Part model, mm, in its own coordinate system. Face numbers are marked on the shaded views. A direction names the side the tool comes from. Coordinates: 2 decimals unless noted, no trailing zeros. Order: outer loops, then holes, each group sorted by start corner. A loop starts at its lowest first (then second) coordinate and runs counter-clockwise, first axis right, second up.
1) Mould opens along X. For the marked faces 1, 2 and 3 say: +X half, -X half, draft (parallel to the pull), parting line (faces both ways), or undercut.
2) Cut at A-A (y = 8.25). List the corners of the cut face in (x, z), and give its area (3 significant figures).
3) Pin check, flat tips, straight feed: pin 1 Ø3 at (y, z) = (4.5, 7) entering from +X; pin 2 Ø3.5 at (x, z) = (-1, -1.5) entering from -Y; pin 3 Ø2 at (x, z) = (-3, 5) entering from -Y. Stop position of each tip, or through.
4) Wall check: L1, parallel to X at y = 13.75, z = 0; L2, parallel to Y at x = -7, z = 3.5; L3, parallel to Y at x = -7.75, z = -1.5. Give the ranges that are in metal, low to high.
5) Tool access for the marked faces 4 and 5: list every direction of +Z, -Z, +X, -X, +Y, -Y with a clear straight run to the whole face (end or side of a thin tool).
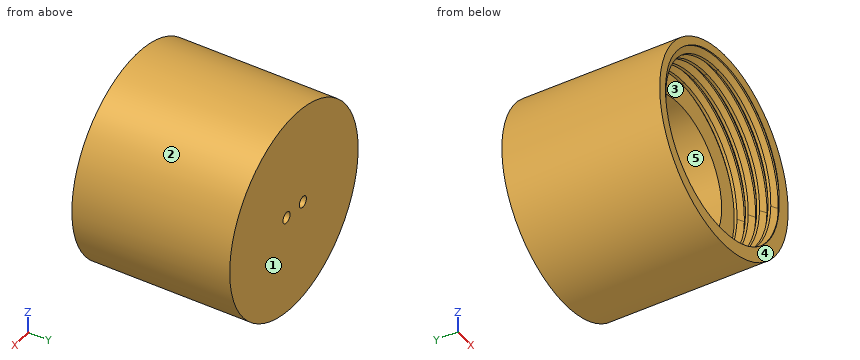
```python
from build123d import *

# Parameters (mm, degrees)
SKETCH1_R           = 9
SKETCH1_R_2         = 7.75
BOSS_EXTRUDE1_DEPTH = 4
SKETCH2_R           = 9
SKETCH2_R_2         = 6
BOSS_EXTRUDE2_DEPTH = 9
THREAD2_PITCH       = 1
THREAD2_TO          = 5
SKETCH3_R           = 9
SKETCH3_R_2         = 0.5
BOSS_EXTRUDE3_DEPTH = 1


with BuildPart() as part:
    # Sketch1 → Boss-Extrude1 (new body)
    with BuildSketch(Plane(origin=(0, 0, 0), x_dir=(1, 0, 0), z_dir=(0, 1, 0))):
        with Locations(Location((0, 0, 0), (0, 0, 270))):
            Circle(SKETCH1_R)
        with Locations(Location((0, 0, 0), (0, 0, 270))):
            Circle(SKETCH1_R_2, mode=Mode.SUBTRACT)
    extrude(amount=BOSS_EXTRUDE1_DEPTH)

    # Sketch2 → Boss-Extrude2 (add)
    with BuildSketch(Plane(origin=(0, 4, 0), x_dir=(1, 0, 0), z_dir=(0, 1, 0))):
        with Locations(Location((0, 0, 0), (0, 0, 270))):
            Circle(SKETCH2_R)
        with Locations(Location((0, 0, 0), (0, 0, 270))):
            Circle(SKETCH2_R_2, mode=Mode.SUBTRACT)
    extrude(amount=BOSS_EXTRUDE2_DEPTH)

    # Thread2: arcs per turn and ends read off the stored shape
    # Thread2: the profile of Thread Profile2 profile screwed along a right-hand helix through 5 turns, 8 arcs to a turn; built about Z, then put on its axis
    thread2_z = Axis((0, 0, 0), (0, 0, 1))
    thread2_corners = [(7.7497, 0, -0.000173205), (8.291265875, 0, 0.312499999), (8.291265875, 0, 0.437499999), (7.7497, 0, 0.750173202)]
    with BuildLine(mode=Mode.PRIVATE) as thread2_profile:
        Line(thread2_corners[0], thread2_corners[1])
        Line(thread2_corners[1], thread2_corners[2])
        Line(thread2_corners[2], thread2_corners[3])
        Line(thread2_corners[3], thread2_corners[0])
    thread2_cap = Face(thread2_profile.wire())
    thread2_turn_angles = [0, 22.5, 45, 67.5, 90, 112.5, 135, 157.5, 180, 202.5, 225, 247.5, 270, 292.5, 315, 337.5, 360]
    thread2_turn_weights = [1, 0.9238795325112867, 1, 0.9238795325112867, 1, 0.9238795325112867, 1, 0.9238795325112867, 1, 0.9238795325112867, 1, 0.9238795325112867, 1, 0.9238795325112867, 1, 0.9238795325112867, 1]
    thread2_turn_rails = [Edge.make_bspline([Vector(p[0], p[1], 0).rotate(thread2_z, thread2_turn_angles[k]) / thread2_turn_weights[k] + Vector(0, 0, p[2] + THREAD2_PITCH * thread2_turn_angles[k] / 360) for k in range(17)], [0, 0, 0, 1, 1, 2, 2, 3, 3, 4, 4, 5, 5, 6, 6, 7, 7, 8, 8, 8], 2, thread2_turn_weights) for p in thread2_corners]
    thread2_turn_sides = [Face.make_surface_from_curves(thread2_turn_rails[p[0]], thread2_turn_rails[p[1]]) for p in [(0, 1), (1, 2), (2, 3), (3, 0)]]
    thread2 = Plane(origin=(0, -1, 0), x_dir=(1, 0, 0), z_dir=(0, 1, 0)) * split(Solid(Shell([*[p.moved(Location((0, 0, THREAD2_PITCH * i))) for i in range(5) for p in thread2_turn_sides], thread2_cap, thread2_cap.rotate(thread2_z, 1800).moved(Location((0, 0, THREAD2_PITCH * 1800 / 360)))])), bisect_by=Plane.XY.offset(THREAD2_TO), keep=Keep.BOTTOM, mode=Mode.PRIVATE)
    add(thread2, mode=Mode.SUBTRACT)

    # Sketch3 → Boss-Extrude3 (add)
    with BuildSketch(Plane(origin=(0, 13, 0), x_dir=(1, 0, 0), z_dir=(0, 1, 0))):
        with Locations(Location((0, 0, 0), (0, 0, 270))):
            Circle(SKETCH3_R)
        with Locations(Location((-1.25, 0, 0), (0, 0, 270))):
            Circle(SKETCH3_R_2, mode=Mode.SUBTRACT)
        with Locations(Location((1.035492966, 0, 0), (0, 0, 270))):
            Circle(SKETCH3_R_2, mode=Mode.SUBTRACT)
    extrude(amount=BOSS_EXTRUDE3_DEPTH)


solid = part.part
```
Geometry check:
1. face 1: draft
1. face 2: parting line
1. face 3: undercut
2. outline: circle Ø18 at (0, 0); hole circle Ø12 at (0, 0)
2. area: 141 mm2
3. pin 1: stops at x = 7.12
3. pin 2: stops at y = 13
3. pin 3: stops at y = 4
4. L1: x = -9 to -1.75, -0.75 to 0.54, 1.54 to 9
4. L2: y = 0.28 to 0.62, 1.28 to 1.62, 2.28 to 2.62, 3.28 to 3.62, 4 to 14
4. L3: y = 0.14 to 0.55, 1.14 to 1.55, 2.14 to 2.55, 3.14 to 3.55, 4 to 14
5. face 4: +Z, -Z, +X, -X, -Y
5. face 5: -Y
